Input: part model. Units: mm. Frame: model coordinates. A direction names the side the tool comes from. Round coordinates to 2 decimals unless told otherwise and drop trailing zeros. Order: outer loops, then holes, each group sorted by start corner. A loop starts at its lowest first (then second) coordinate and runs counter-clockwise, first axis right, second up.
Item 1: Reachability of faces 1 (the flat face through (0, 67, 6.35)), 2 (the cylindrical face through (-3, 4, 0)) from +Z, -Z, +X, -X, +Y, -Y: full face, straight path, thin tool, end or side. Return the list, or none.
Item 2: Cut plane A-A on x = 0. Output: boundary loops of the cut face in (y, z).
Item 3: Cut plane D-D on x = 4.75. Output: boundary loops of the cut face in (y, z), then the cut area to 3 significant figures.
Item 4: Cut plane B-B on y = 40. Output: boundary loops of the cut face in (x, z), then the cut area to 3 significant figures.
Item 5: Cut plane C-C on z = 1.75. Output: boundary loops of the cut face in (x, y), then the cut area to 3 significant figures.
Item 6: First-contact query: pin 1 (1.5 mm diameter, centred on x = 4.5, z = -1.5, fed in from -Y); pin 2 (1.5 mm diameter, centred on y = 78.5, z = -3.5, fed in from -X). Flat tips, straight axial feed; report the tip coordinate or a pass-through.
Item 7: Line query: L1, parallel to Y at x = 0.75, z = -3.75; L2, parallel to X at y = 83, z = 2; L3, parallel to X at y = 75.5, z = -4.75. Output: solid intervals per line, ascending.
```python
from build123d import *

# Parameters (mm, degrees)
BOSS_EXTRUDE1_DEPTH = 127
SKETCH3_R           = 18.31161494
SKETCH3_R_2         = 3
CUT_EXTRUDE1_DEPTH  = 8.5


with BuildPart() as part:
    # Sketch1 → Boss-Extrude1 (new body)
    with BuildSketch(Plane(origin=(0, 0, 0), x_dir=(1, 0, 0), z_dir=(0, 1, 0))):
        Polygon((7.332348419, 0), (3.666174209, 6.35), (-3.666174209, 6.35), (-7.332348419, 0), (-3.666174209, -6.35), (3.666174209, -6.35), align=None)
    extrude(amount=BOSS_EXTRUDE1_DEPTH)

    # Sketch3 → Cut-Extrude1 (cut)
    with BuildSketch(Plane.XZ):
        Circle(SKETCH3_R)
        Circle(SKETCH3_R_2, mode=Mode.SUBTRACT)
    extrude(amount=-CUT_EXTRUDE1_DEPTH, mode=Mode.SUBTRACT)


solid = part.part
```
From the geometry:
1. face 1: +Z, +X, -X, +Y, -Y
1. face 2: -Y
2. outline: (0, -3) - (8.5, -3) - (8.5, -6.35) - (127, -6.35) - (127, 6.35) - (8.5, 6.35) - (8.5, 3) - (0, 3) - close
3. outline: (8.5, -4.47) - (127, -4.47) - (127, 4.47) - (8.5, 4.47) - close
3. area: 1,060 mm2
4. outline: (-7.33, 0) - (-3.67, -6.35) - (3.67, -6.35) - (7.33, 0) - (3.67, 6.35) - (-3.67, 6.35) - close
4. area: 140 mm2
5. outline: (-6.32, 8.5) - (-2.44, 8.5) - (-2.44, 0) - (2.44, 0) - (2.44, 8.5) - (6.32, 8.5) - (6.32, 127) - (-6.32, 127) - close
5. area: 1,540 mm2
6. pin 1: stops at y = 8.5
6. pin 2: stops at x = -5.74
7. L1: y = 8.5 to 127
7. L2: x = -6.18 to 6.18
7. L3: x = -4.59 to 4.59
